CAD build for the part. Positions are in the model's coordinates, mm. A direction names the side the tool comes from. Give positions to 0.01 mm unless a question says otherwise; leave off trailing zeros. Write each loop counter-clockwise with the first axis right and the second up, starting at its lowest first coordinate (ties: lowest second). Pieces come first, ordered by that corner, then holes. Notation, with made-up numbers: (20.25, -12) - (56.25, -12) arc R17 cw to (56.25, -7) - close; hole circle Ø11 at (18, -30.5). An arc over 180 degrees is marked (long way). Answer as a JSON object with one key per item and string values.
from build123d import *

# Parameters (mm, degrees)
SKETCH1_W           = 40
SKETCH1_H           = 20
SKETCH1_R           = 1.75
BOSS_EXTRUDE1_DEPTH = 2.4
SKETCH2_W           = 40
SKETCH2_H           = 5
BOSS_EXTRUDE2_DEPTH = 5.5
FILLET1_R           = 2


with BuildPart() as part:
    # Sketch1 → Boss-Extrude1 (new body)
    with BuildSketch(Plane(origin=(0, 0, 0), x_dir=(1, 0, 0), z_dir=(0, 1, 0))):
        with Locations((20, 10)):
            Rectangle(SKETCH1_W, SKETCH1_H)
        with Locations((10, 10)):
            Circle(SKETCH1_R, mode=Mode.SUBTRACT)
        with Locations((30, 10)):
            Circle(SKETCH1_R, mode=Mode.SUBTRACT)
    extrude(amount=BOSS_EXTRUDE1_DEPTH)

    # Sketch2 → Boss-Extrude2 (add)
    with BuildSketch(Plane(origin=(0, 2.4, 0), x_dir=(1, 0, 0), z_dir=(0, 1, 0))):
        with Locations((20, -2.5)):
            Rectangle(SKETCH2_W, SKETCH2_H)
    extrude(amount=-BOSS_EXTRUDE2_DEPTH)

    # Fillet1
    fillet1_edges = [part.edges().sort_by_distance(p)[0] for p in [
        (20, 2.4, 5),
    ]]
    fillet(fillet1_edges, radius=FILLET1_R)


solid = part.part
Item 1: Mould opens along X. For faces 1 (the flat face through (20, -1, 5)), 2 (the cylindrical face through (10.9, 1.2, -11.5)), 3 (the flat face through (40, 1, -5)) say: +X half, -X half, draft (parallel to the pull), parting line (faces both ways), or undercut.
Entries:
{"face 1": "draft", "face 2": "undercut", "face 3": "+X half"}
Item 2: Cut at C-C (x = 34). Give the cut face in (y, z).
Entries:
{"outline": "(-3.1, 0) - (0, 0) - (0, -20) - (2.4, -20) - (2.4, 3) arc R2 ccw to (0.4, 5) - (-3.1, 5) - close"}
Item 3: Cut at A-A (z = -10). Give the cut face in (x, y).
Entries:
{"outline": "(0, 0) - (8.25, 0) - (8.25, 2.4) - (0, 2.4) - close; (11.75, 0) - (28.25, 0) - (28.25, 2.4) - (11.75, 2.4) - close; (31.75, 0) - (40, 0) - (40, 2.4) - (31.75, 2.4) - close"}
Item 4: Which spindle directions (+Z, -Z, +X, -X, +Y, -Y) get a long thin tool onto all of the face, cutting with end or side? Do faces 4 (the flat face through (20, 1, -20)), 5 (the flat face through (20, 0, -10)). Say none if no direction does.
Entries:
{"face 4": "-Z, +X, -X, +Y, -Y", "face 5": "-Z, +X, -X, -Y"}
Item 5: Cut at D-D (y = 1). Give the cut face in (x, z).
Entries:
{"outline": "(0, -20) - (40, -20) - (40, 4.91) - (0, 4.91) - close; hole circle Ø3.5 at (10, -10); hole circle Ø3.5 at (30, -10)"}
Item 6: Cut at B-B (x = 30). Give the cut face in (y, z).
Entries:
{"outline": "(-3.1, 0) - (0, 0) - (0, -8.25) - (2.4, -8.25) - (2.4, 3) arc R2 ccw to (0.4, 5) - (-3.1, 5) - close; (0, -20) - (2.4, -20) - (2.4, -11.75) - (0, -11.75) - close"}
Item 7: Flat gauge pins, fed straight in: P1, Ø1, axis at y = 1.5, z = -17.5, coming from the -X side; P2, Ø3, axis at x = 30, z = -10, coming from the -Y side; P3, Ø2.5, axis at x = 27.5, y = -2.5, coming from the -Z side; P4, Ø3, axis at x = 18, z = -14.5, coming from the -Y side. Where does each tip first touch, or does it go through?
Entries:
{"P1": "x = 0", "P2": "through", "P3": "z = 0", "P4": "y = 0"}
Item 8: Probe line 1 (X direction, y = 0.85, z = -10); line 2 (X direction, y = 1.05, z = -8.75); line 3 (Y direction, x = 10.5, z = -6.75). List the from-to ranges inside material, lowest first. Write a range as from..to.
Entries:
{"line 1": "0..8.25, 11.75..28.25, 31.75..40", "line 2": "0..8.78, 11.22..28.78, 31.22..40", "line 3": "0..2.4"}
